from build123d import *

# Parameters (mm, degrees)
F0_W     = 57.15
F0_H     = 57.15
F1_DEPTH = 9.525
F2_R     = 19.177
F3_DEPTH = 6.35
F4_R     = 2.413
F5_DEPTH = 9.526
F7_R     = 4.191
F8_DEPTH = 9.526
F6_R     = 5.842
F9_DEPTH = 6.35
F10_SIZE = 6.35


with BuildPart() as f1:
    # F0 (on Top) → F1 (new body)
    with BuildSketch(Plane.XY):
        Rectangle(F0_W, F0_H)
    extrude(amount=F1_DEPTH)

    # F2 (on face) → F3 (cut)
    with BuildSketch(Plane.XY.offset(9.525)):
        Circle(F2_R)
    extrude(amount=-F3_DEPTH, mode=Mode.SUBTRACT)

    # F4 (on Top) → F5 (cut, through all)
    with BuildSketch(Plane.XY):
        with Locations((-19.05, 19.050001)):
            Circle(F4_R)
        with Locations((19.05, 19.050001)):
            Circle(F4_R)
        with Locations((-19.05, -19.050001)):
            Circle(F4_R)
        with Locations((19.05, -19.050001)):
            Circle(F4_R)
    extrude(amount=F5_DEPTH, mode=Mode.SUBTRACT)

    # F7 (on Top) → F8 (cut, through all)
    with BuildSketch(Plane.XY):
        with Locations((0, 8.255)):
            Circle(F7_R)
        with Locations((0, -8.255)):
            Circle(F7_R)
    extrude(amount=F8_DEPTH, mode=Mode.SUBTRACT)

    # F6 (on face) → F9 (cut)
    with BuildSketch(Plane.XY.offset(9.525)):
        with Locations((-19.05, 19.050001)):
            Circle(F6_R)
        with Locations((19.05, 19.050001)):
            Circle(F6_R)
        with Locations((-19.05, -19.050001)):
            Circle(F6_R)
        with Locations((19.05, -19.050001)):
            Circle(F6_R)
    extrude(amount=-F9_DEPTH, mode=Mode.SUBTRACT)

    # F10
    f10_edges = [f1.edges().sort_by_distance(p)[0] for p in [
        (-28.575, -28.575, 4.7625),
        (28.575, -28.575, 4.7625),
        (28.575, 28.575, 4.7625),
        (-28.575, 28.575, 4.7625),
    ]]
    chamfer(f10_edges, length=F10_SIZE)


solid = f1.part
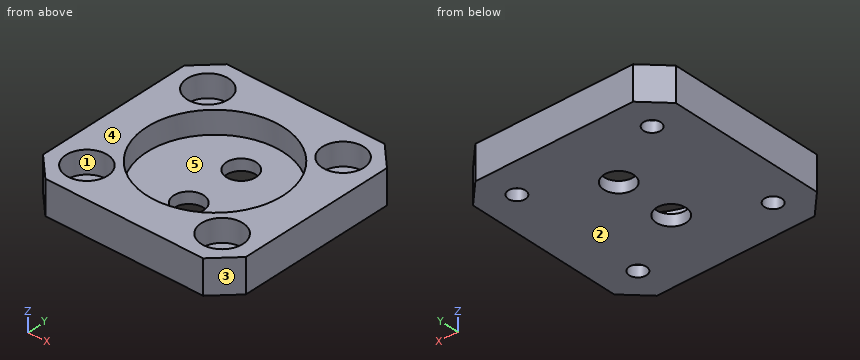
The listing builds one solid part. Answer for the finished solid, in the listing's coordinates (mm). Face numbers are marked on the shaded views. A direction names the side the tool comes from. Give positions to 0.01 mm unless a question says otherwise; leave off trailing zeros. Write each loop counter-clockwise with the first axis right and the second up, starting at its lowest first coordinate (ties: lowest second). Pieces come first, ordered by that corner, then holes.
1) Section D-D (z = 2.25) is taken. Write down the section's boundary in (x, y) (3 decimals), and give its area (3 significant figures).
2) A tool of negligible diameter and unlimited length cuts with its end or side. For the marked faces 4 and 5, from which of +Z, -Z, +X, -X, +Y, -Y can it reach the whole face along a straight path? Write none if from no direction.
3) Find the intervals of material crossed by L1, parallel to Y at x = 0, z = 0.7 (3 decimals); L2, parallel to X at y = 19, z = 2.25 (3 decimals); L3, parallel to X at y = -21, z = 9 (3 decimals), in increasing order.
4) Given P1, Ø1, axis at x = -17.5, y = 1, coming from the +Z side (3 decimals), flat-ended and moving along its own axis, determine where the tip first touches the part or whether it passes through.
5) Section C-C (z = 7) is taken. Write down the section's boundary in (x, y) (3 decimals).
6) For a pull along X with two mould halves and no side action, classify the marked faces 1, 2 and 3 as pulls with the +X half, pulls with the -X half, needs draft (parallel to the pull), parting line crosses it, or undercut.
7) Section A-A (x = 0) is taken. Write down the section's boundary in (y, z) (3 decimals).
8) Section B-B (y = 0) is taken. Write down the section's boundary in (x, z) (3 decimals), and give its area (3 significant figures).
Response:
1. outline: (-28.575, -22.225) - (-22.225, -28.575) - (22.225, -28.575) - (28.575, -22.225) - (28.575, 22.225) - (22.225, 28.575) - (-22.225, 28.575) - (-28.575, 22.225) - close; hole circle Ø4.826 at (-19.05, -19.05); hole circle Ø4.826 at (-19.05, 19.05); hole circle Ø8.382 at (0, -8.255); hole circle Ø8.382 at (0, 8.255); hole circle Ø4.826 at (19.05, -19.05); hole circle Ø4.826 at (19.05, 19.05)
1. area: 3,000 mm2
2. face 4: +Z, +X, -X, +Y, -Y
2. face 5: +Z
3. L1: y = -28.575 to -12.446, -4.064 to 4.064, 12.446 to 28.575
3. L2: x = -28.575 to -21.462, -16.638 to 16.638, 21.462 to 28.575
3. L3: x = -28.575 to -24.557, -13.543 to 13.543, 24.557 to 28.575
4. P1: stops at z = 3.175
5. outline: (-28.575, -22.225) - (-22.225, -28.575) - (22.225, -28.575) - (28.575, -22.225) - (28.575, 22.225) - (22.225, 28.575) - (-22.225, 28.575) - (-28.575, 22.225) - close; hole circle Ø11.684 at (-19.05, -19.05); hole circle Ø11.684 at (-19.05, 19.05); hole circle Ø38.354 at (0, 0); hole circle Ø11.684 at (19.05, -19.05); hole circle Ø11.684 at (19.05, 19.05)
6. face 1: undercut
6. face 2: needs draft
6. face 3: pulls with the +X half
7. outline: (-28.575, 0) - (-12.446, 0) - (-12.446, 3.175) - (-19.177, 3.175) - (-19.177, 9.525) - (-28.575, 9.525) - close; (-4.064, 0) - (4.064, 0) - (4.064, 3.175) - (-4.064, 3.175) - close; (12.446, 0) - (28.575, 0) - (28.575, 9.525) - (19.177, 9.525) - (19.177, 3.175) - (12.446, 3.175) - close
8. outline: (-28.575, 0) - (28.575, 0) - (28.575, 9.525) - (19.177, 9.525) - (19.177, 3.175) - (-19.177, 3.175) - (-19.177, 9.525) - (-28.575, 9.525) - close
8. area: 301 mm2
